For this review, use the dimensioned drawing (mm, ordinates from the lowest corner) and the shaded views. A direction names the side the tool comes from. Coordinates: 2 decimals unless noted, no trailing zeros. Loops run counter-clockwise (first coordinate to the right, second up) from the corner with the lowest first, then second, coordinate; pieces in that order, holes last. Notation, with made-up numbers: (-13, -17) - (10, -17) arc R13 ccw to (10, 3) - close; hole circle Ø2 at (15, -26). An arc over 180 degrees is marked (long way). Answer in a Markdown table with one row per item. Add a question column.
(1) We need section B-B on z = 5.25. Write out the cut boundary in (x, y), plus the area to 3 significant figures.
(2) Mouldability with a two-part tool opening along X and no side actions: class the marked faces 1, 2 and 3 as +X half, -X half, draft (parallel to the pull), parting line (faces both ways), or undercut.
(3) For line 1 along Y through (x, z) = (20.5, 7.75); line 2 along X through (y, z) = (14, 10); line 3 along X through (y, z) = (2.75, 11), list the stretches that pass through material, from the lowest coordinate up.
(4) We need section D-D on y = 13.5. Write out the cut boundary in (x, z), plus the area to 3 significant figures.
(5) For P1, Ø5, axis at x = 33.5, z = 2, coming from the -Y side; P2, Ø1.5, axis at x = 42, y = 1.5, coming from the -Z side; P3, Ø6, axis at x = 21, z = 9, coming from the -Y side; P4, Ø1, axis at x = 29.5, z = 13, coming from the +Y side, all flat-tipped, find the tip position at first contact; note any pin that passes through.
(6) We need section A-A on y = 2.25. Write out the cut boundary in (x, z).
(7) Machinability: for the marked faces 4, 5 and 6, which of the approach directions +Z, -Z, +X, -X, +Y, -Y give a long, thin tool a straight path to every point of the face, cutting with its end or side? Answer none if there is none.
(8) We need section C-C on x = 22. Write out the cut boundary in (y, z), plus the area to 3 significant figures.
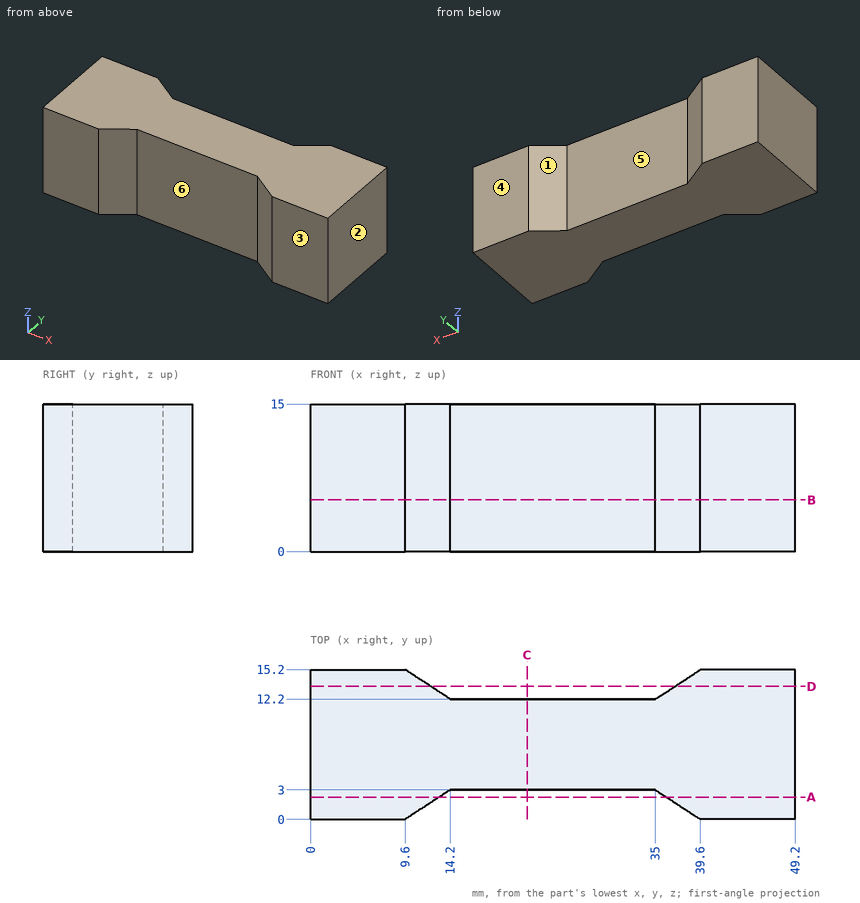
Outcome:
| question | item | result |
|---|---|---|
| 1 | outline | (0, 0) - (9.6, 0) - (14.2, 3) - (35, 3) - (39.6, 0) - (49.2, 0) - (49.2, 15.2) - (39.6, 15.2) - (35, 12.2) - (14.2, 12.2) - (9.6, 15.2) - (0, 15.2) - close |
| 1 | area | 595 mm² |
| 2 | face 1 | undercut |
| 2 | face 2 | +X half |
| 2 | face 3 | draft |
| 3 | line 1 | 3 to 12.2 |
| 3 | line 2 | 0 to 11.44, 37.76 to 49.2 |
| 3 | line 3 | 0 to 13.82, 35.38 to 49.2 |
| 4 | outline | (0, 0) - (12.21, 0) - (12.21, 15) - (0, 15) - close; (36.99, 0) - (49.2, 0) - (49.2, 15) - (36.99, 15) - close |
| 4 | area | 366 mm² |
| 5 | P1 | y = 2.35 |
| 5 | P2 | z = 0 |
| 5 | P3 | y = 3 |
| 5 | P4 | y = 12.2 |
| 6 | outline | (0, 0) - (13.05, 0) - (13.05, 15) - (0, 15) - close; (36.15, 0) - (49.2, 0) - (49.2, 15) - (36.15, 15) - close |
| 7 | face 4 | +Z, -Z, +X, -X, +Y |
| 7 | face 5 | +Z, -Z, +Y |
| 7 | face 6 | +Z, -Z, -Y |
| 8 | outline | (3, 0) - (12.2, 0) - (12.2, 15) - (3, 15) - close |
| 8 | area | 138 mm² |
